Verification items for the finished model (mm, model axes). Face numbers are marked on the shaded views. Round coordinates to 2 decimals unless told otherwise and drop trailing zeros. Write each loop counter-clockwise with the first axis right and the second up, starting at its lowest first coordinate (ties: lowest second). Pieces come first, ordered by that corner, then holes. Notation, with made-up numbers: M 80,24 L 119,24 A13 cw 119,44 Z; hole C 68.5,37.25 d2. An arc over 180 degrees is marked long. Write each question's results on one line, items separated by ' | '.
from build123d import *

# Parameters (mm, degrees)
F0_R     = 9.5
F0_R_2   = 7.5
F1_DEPTH = 40
F2_R     = 9.5
F2_R_2   = 7.5
F3_DEPTH = 15
F4_R     = 7.5
F5_DEPTH = 50
F6_R     = 7.5
F7_DEPTH = 15


with BuildPart() as f1:
    # F0 (on Right) → F1 (new body)
    with BuildSketch(Plane.YZ):
        Circle(F0_R)
        Circle(F0_R_2, mode=Mode.SUBTRACT)
    extrude(amount=F1_DEPTH)

    # F2 (on Top) → F3 (join)
    with BuildSketch(Plane.XY):
        with Locations((20, 0)):
            Circle(F2_R)
        with Locations((20, 0)):
            Circle(F2_R_2, mode=Mode.SUBTRACT)
    extrude(amount=F3_DEPTH)

    # F4 (on face) → F5 (cut)
    with BuildSketch(Plane.YZ.offset(40)):
        Circle(F4_R)
    extrude(amount=-F5_DEPTH, mode=Mode.SUBTRACT)

    # F6 (on face) → F7 (cut)
    with BuildSketch(Plane.XY.offset(15)):
        with Locations((20, 0)):
            Circle(F6_R)
    extrude(amount=-F7_DEPTH, mode=Mode.SUBTRACT)


solid = f1.part
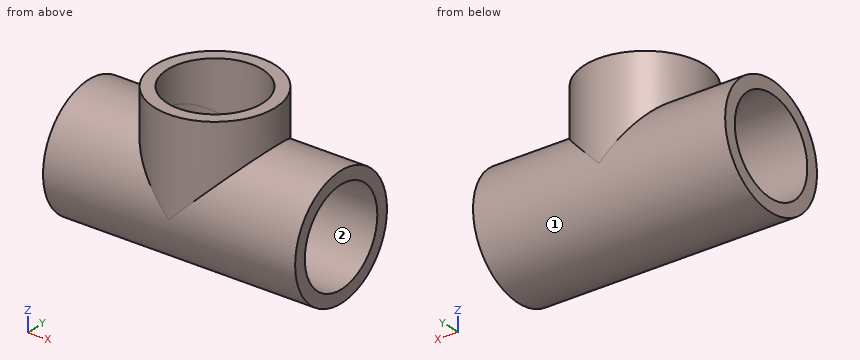
1) Draft check along Z on the marked faces 1 and 2. Enter one of: pulls with the +Z half, pulls with the -Z half, needs draft (parallel to the pull), parting line crosses it, or undercut.
Calculated:
face 1: parting line crosses it | face 2: undercut
2) Sectioned sample at B-B, the plane z = -5. Record the cut outline in (x, y).
Calculated:
outline: M 0,-8.08 L 40,-8.08 L 40,-5.59 L 0,-5.59 Z; M 0,5.59 L 40,5.59 L 40,8.08 L 0,8.08 Z
3) Sectioned sample at D-D, the plane z = 12.5. Record the cut outline in (x, y).
Calculated:
outline: C 20,0 d19; hole C 20,0 d15
4) Sectioned sample at A-A, the plane y = 0. Record the cut outline in (x, z), and give its area (3 significant figures).
Calculated:
outline: M 0,-9.5 L 40,-9.5 L 40,-7.5 L 0,-7.5 Z; M 0,7.5 L 12.5,7.5 L 12.5,15 L 10.5,15 L 10.5,9.5 L 0,9.5 Z; M 27.5,7.5 L 40,7.5 L 40,9.5 L 29.5,9.5 L 29.5,15 L 27.5,15 Z | area: 152 mm²
5) Depth check by flat-ended pin: P1, Ø6, axis at x = 10, z = 5, coming from the -Y side; P2, Ø5, axis at y = -6.5, z = 1, coming from the +X side; P3, Ø9, axis at x = 20, y = 0, coming from the +Z side; P4, Ø2, axis at x = 17.5, y = 4, coming from the +Z side. Enter the tip coordinate at first touch or a pass-through.
Calculated:
P1: stops at y = -9.29 | P2: stops at x = 40 | P3: stops at z = -6 | P4: stops at z = -5.59
6) Material ranges on line 1 (X direction, y = 0, z = 12.25); line 2 (Y direction, x = 28.5, z = 0), recorded low to high. Write a range as [from, to].
Calculated:
line 1: x = [10.5, 12.5], [27.5, 29.5] | line 2: y = [-9.5, -7.5], [7.5, 9.5]
7) Sectioned sample at C-C, the plane x = 20. Record the cut outline in (y, z), and give its area (3 significant figures).
Calculated:
outline: M -9.5,0 A9.5 ccw 9.5,0 L 9.5,15 L 7.5,15 L 7.5,0 A7.5 cw -7.5,0 L -7.5,15 L -9.5,15 Z | area: 113 mm²
